Here's how the part is built. I have some questions about the finished solid (model axes, mm). A direction names the side the tool comes from. Round coordinates to 2 decimals unless told otherwise and drop trailing zeros. Write each loop counter-clockwise with the first axis right and the second up, starting at its lowest first coordinate (ties: lowest second). Pieces come first, ordered by that corner, then holes. Notation, with made-up numbers: (12.25, -6.5) -> (20.25, -6.5) arc R11 ccw to (20.25, 13.5) -> close; hole circle Ø4 at (70.5, -6). An arc over 180 degrees is marked (long way). Answer as CSV lines item,"result".
from build123d import *

# Parameters (mm, degrees)
SKETCH046_R          = 60
PAD019_DEPTH         = 45
SKETCH047_R          = 54.5
POCKET020_DEPTH      = 40.5
SKETCH054_W          = 13.996185
SKETCH054_H          = 10.514995
POCKET022_DEPTH      = 3
SKETCH055_W          = 3.607353
SKETCH055_H          = 10.482647
POCKET023_DEPTH      = 46.501
SKETCH056_W          = 22.63
SKETCH056_H          = 10.08
POCKET024_DEPTH      = 5
SKETCH058_R          = 3.35
POCKET025_DEPTH      = 5
POCKET025_DEPTH_BACK = 100
SKETCH059_R          = 57
POCKET026_DEPTH      = 10
SKETCH061_W          = 15
SKETCH061_H          = 29
PAD028_DEPTH         = 26.5
SKETCH062_W          = 12.44
SKETCH062_H          = 22.8
POCKET027_DEPTH      = 12.5
POCKET027_DEPTH_BACK = 6
SKETCH063_W          = 11.698539
SKETCH063_H          = 10.75206
POCKET031_DEPTH      = 5
POCKET032_DEPTH      = 18.28
SKETCH070_W          = 5.148875
SKETCH070_H          = 8.518356
POCKET033_DEPTH      = 5


with BuildPart() as part:
    # Sketch046 → Pad019 (new body)
    with BuildSketch(Plane.XZ):
        with Locations((52.5, -52.5)):
            Circle(SKETCH046_R)
    extrude(amount=PAD019_DEPTH)

    # Sketch047 (on Face2 of Pad019) → Pocket020 (cut)
    with BuildSketch(Plane(origin=(0, 0, 0), x_dir=(1, 0, 0), z_dir=(0, 1, 0))):
        with Locations((52.5, 52.5)):
            Circle(SKETCH047_R)
    extrude(amount=-POCKET020_DEPTH, mode=Mode.SUBTRACT)

    # Sketch054 → Pocket022 (cut)
    with BuildSketch(Plane.XZ.offset(52.5)):
        with Locations((89.9295195, -51.4149685)):
            Rectangle(SKETCH054_W, SKETCH054_H)
    extrude(amount=-POCKET022_DEPTH, mode=Mode.SUBTRACT)

    # Sketch055 (on Face37 of Pocket022) → Pocket023 (cut, through all)
    with BuildSketch(Plane.XZ.offset(46.5)):
        with Locations((84.7541845, -51.4075485)):
            Rectangle(SKETCH055_W, SKETCH055_H)
    extrude(amount=-POCKET023_DEPTH, mode=Mode.SUBTRACT)

    # Sketch056 (on Face3 of Pocket023) → Pocket024 (cut)
    with BuildSketch(Plane.XZ.offset(45)):
        with Locations((52.3097458031, -95.0004416785)):
            Rectangle(SKETCH056_W, SKETCH056_H)
    extrude(amount=-POCKET024_DEPTH, mode=Mode.SUBTRACT)

    # Sketch058 → Pocket025 (cut, two sides)
    with BuildSketch(Plane(origin=(0, -44.5, 0), x_dir=(1, 0, 0), z_dir=(0, 1, 0))) as pocket025_sk:
        with Locations((16.6674273862, 50.4959887414)):
            Circle(SKETCH058_R)
    extrude(amount=-POCKET025_DEPTH, mode=Mode.SUBTRACT)
    extrude(pocket025_sk.sketch, amount=POCKET025_DEPTH_BACK, mode=Mode.SUBTRACT)

    # Sketch059 (on Face2 of Pocket025) → Pocket026 (cut)
    with BuildSketch(Plane(origin=(0, 0, 0), x_dir=(1, 0, 0), z_dir=(0, 1, 0))):
        with Locations((52.5, 52.5)):
            Circle(SKETCH059_R)
    extrude(amount=-POCKET026_DEPTH, mode=Mode.SUBTRACT)

    # Sketch061 (on Face15 of Pocket026) → Pad028 (join)
    with BuildSketch(Plane(origin=(0, -40.5, 0), x_dir=(1, 0, 0), z_dir=(0, 1, 0))):
        with Locations((52.5, 52.5)):
            Rectangle(SKETCH061_W, SKETCH061_H)
    extrude(amount=PAD028_DEPTH)

    # Sketch062 → Pocket027 (cut, two sides)
    with BuildSketch(Plane(origin=(0, -20, 0), x_dir=(1, 0, 0), z_dir=(0, 1, 0))) as pocket027_sk:
        with Locations((52.5, 52.5)):
            Rectangle(SKETCH062_W, SKETCH062_H)
    extrude(amount=-POCKET027_DEPTH, mode=Mode.SUBTRACT)
    extrude(pocket027_sk.sketch, amount=POCKET027_DEPTH_BACK, mode=Mode.SUBTRACT)

    # Sketch063 (on Face18 of Pocket027) → Pocket031 (cut)
    with BuildSketch(Plane(origin=(0, 0, -38), x_dir=(-1, 0, 0), z_dir=(0, 0, 1))):
        with Locations((-52.4716495, 26.589729)):
            Rectangle(SKETCH063_W, SKETCH063_H)
    extrude(amount=-POCKET031_DEPTH, mode=Mode.SUBTRACT)

    # Sketch064 (on Face17 of Pocket031) → Pocket032 (cut)
    with BuildSketch(Plane(origin=(45, 0, 0), x_dir=(0, 0, -1), z_dir=(-1, 0, 0))):
        Polygon((48.289669, 29.4052434227), (46.789669, 32.0033196341), (43.789669, 32.0033196341), (42.289669, 29.4052434227), (43.789669, 26.8071672114), (46.789669, 26.8071672114), align=None)
        Polygon((48.289669, 23.209091), (46.789669, 25.8071672114), (43.789669, 25.8071672114), (42.289669, 23.209091), (43.789669, 20.6110147886), (46.789669, 20.6110147886), align=None)
        Polygon((55.289669, 29.4052434227), (53.789669, 32.0033196341), (50.789669, 32.0033196341), (49.289669, 29.4052434227), (50.789669, 26.8071672114), (53.789669, 26.8071672114), align=None)
        Polygon((55.289669, 23.209091), (53.789669, 25.8071672114), (50.789669, 25.8071672114), (49.289669, 23.209091), (50.789669, 20.6110147886), (53.789669, 20.6110147886), align=None)
        Polygon((62.289669, 29.4052434227), (60.789669, 32.0033196341), (57.789669, 32.0033196341), (56.289669, 29.4052434227), (57.789669, 26.8071672114), (60.789669, 26.8071672114), align=None)
        Polygon((62.289669, 23.209091), (60.789669, 25.8071672114), (57.789669, 25.8071672114), (56.289669, 23.209091), (57.789669, 20.6110147886), (60.789669, 20.6110147886), align=None)
        Polygon((48.289669, 17.0129385773), (46.789669, 19.6110147886), (43.789669, 19.6110147886), (42.289669, 17.0129385773), (43.789669, 14.4148623659), (46.789669, 14.4148623659), align=None)
        Polygon((55.289669, 17.0129385773), (53.789669, 19.6110147886), (50.789669, 19.6110147886), (49.289669, 17.0129385773), (50.789669, 14.4148623659), (53.789669, 14.4148623659), align=None)
        Polygon((62.289669, 17.0129385773), (60.789669, 19.6110147886), (57.789669, 19.6110147886), (56.289669, 17.0129385773), (57.789669, 14.4148623659), (60.789669, 14.4148623659), align=None)
    extrude(amount=-POCKET032_DEPTH, mode=Mode.SUBTRACT)

    # Sketch070 (on Face167 of Pad029) → Pocket033 (cut)
    with BuildSketch(Plane(origin=(0, 0, -41.1), x_dir=(1, 0, 0), z_dir=(0, 0, -1))):
        with Locations((52.6262685, 17.84922)):
            Rectangle(SKETCH070_W, SKETCH070_H)
    extrude(amount=-POCKET033_DEPTH, mode=Mode.SUBTRACT)


with BuildPart() as part_1:
    # Body008 placement: moved
    add(part.part.moved(Location((0, 155, 0))))


solid = part_1.part
Item 1: For faces 1 (the flat face through (57, 133.786, -40)), 2 (the flat face through (46, 141, -54)), 3 (the flat face through (86.558, 112, -51)), which set-ups out of +Z, -Z, +X, -X, +Y, -Y let a thin tool reach every point of the face, with its end or its side?
Results found:
face 1,"none"
face 2,"+Y"
face 3,"+Y, -Y"
Item 2: Suppose I cut it at A-A, the plane x = 52.5. List the corners of the cut face in (y, z) for me, then the cut area to 3 significant figures.
Results found:
outline,"(110, -112.5) -> (155, -112.5) -> (155, -109.5) -> (145, -109.5) -> (145, -107) -> (114.5, -107) -> (114.5, -100.04) -> (110, -100.04) -> close; (110, -89.96) -> (114.5, -89.96) -> (114.5, -67) -> (141, -67) -> (141, -63.9) -> (122.5, -63.9) -> (122.5, -41.1) -> (123.03, -41.1) -> (123.03, -38) -> (114.5, -38) -> (114.5, 2) -> (145, 2) -> (145, 4.5) -> (155, 4.5) -> (155, 7.5) -> (110, 7.5) -> close"
area,"1,180 mm²"
Item 3: Suppose I cut it at B-B, the plane z = -98. List the corners of the cut face in (x, y) for me, then the cut area to 3 significant figures.
Results found:
outline,"(13.39, 110) -> (40.99, 110) -> (40.99, 114.5) -> (22.5, 114.5) -> (22.5, 145) -> (18.17, 145) -> (18.17, 155) -> (13.39, 155) -> close; (63.62, 110) -> (91.61, 110) -> (91.61, 155) -> (86.83, 155) -> (86.83, 145) -> (82.5, 145) -> (82.5, 114.5) -> (63.62, 114.5) -> close"
area,"902 mm²"
Item 4: I need wall thicknesses on L1, parallel to Z at x = 52, y = 131; L2, parallel to X at y = 121, z = -53.5; L3, parallel to Z at x = 52.5, y = 152.75. Which ranges of each line are inside material? Lowest first, please.
Results found:
L1,"z = -112.5 to -107, -67 to -63.9, 2 to 7.5"
L2,"x = -7.49 to -1.99, 45 to 60, 106.99 to 112.49"
L3,"z = -112.5 to -109.5, 4.5 to 7.5"
Item 5: If we mould it in two halves opening along X, with no side actions, what happens to faces 4 (the cylindrical face through (105.154, 150.07, -30.669)), 5 (the flat face through (52, 110, -52))? For each: pulls with the +X half, pulls with the -X half, needs draft (parallel to the pull), parting line crosses it, or undercut.
Results found:
face 4,"undercut"
face 5,"needs draft"
Item 6: Will these pins go through, and if not, where does the flat tip stop? pin 1 (4 mm diameter, centred on x = 27, y = 122, fed in from +Z); pin 2 (6 mm diameter, centred on x = 17, y = 149.5, fed in from +Z); pin 3 (12 mm diameter, centred on x = 36.5, y = 149, fed in from -Z); pin 4 (20.5 mm diameter, centred on y = 131.5, z = -55.5, fed in from -X).
Results found:
pin 1,"stops at z = 2.71"
pin 2,"stops at z = -2.06"
pin 3,"stops at z = -111.66"
pin 4,"stops at x = -7.5"
Item 7: Suppose I cut it at C-C, the plane y = 150. List the corners of the cut face in (x, z) for me.
Results found:
outline,"circle Ø120 at (52.5, -52.5); hole circle Ø114 at (52.5, -52.5)"
Item 8: Suppose I cut it at D-D, the plane z = -22.5. List the corners of the cut face in (x, y) for me, then the cut area to 3 significant figures.
Results found:
outline,"(0.54, 110) -> (104.46, 110) -> (104.46, 155) -> (100.97, 155) -> (100.97, 145) -> (98, 145) -> (98, 114.5) -> (7, 114.5) -> (7, 145) -> (4.03, 145) -> (4.03, 155) -> (0.54, 155) -> close"
area,"932 mm²"
